The listing builds one solid part. Answer for the finished solid, in the listing's coordinates (mm). A direction names the side the tool comes from. Round coordinates to 2 decimals unless told otherwise and drop trailing zeros. Loops run counter-clockwise (first coordinate to the right, second up) from the corner with the lowest first, then second, coordinate; pieces in that order, holes last. Notation, with made-up numbers: (-31, 29) - (-3, 29) arc R11 ccw to (-3, 40) - close; hole circle Ø10 at (-16.75, -6). An arc over 180 degrees is marked (long way). Write item = value, one per line. Start each with the question number.
1) For a pull along X with two mould halves and no side action, classify faces 4 (the cylindrical face through (24.4, 2.97, 28.21)), 5 (the cylindrical face through (-271.8, 4.9, 56.4)), 6 (the flat face through (-358, 5, 41)), 7 (the flat face through (32, 5, 41)) as released by +X, released by -X, zero draft, split by the parting line, or undercut.
2) Given pin 1 Ø5 at (y, z) = (5, 56) entering from +X, flat-ended and moving along its own axis, determine where the tip first touches the part or whether it passes through.
3) A tool of negligible diameter and unlimited length cuts with its end or side. For faces 1 (the cylindrical face through (24, 5, 59)), 2 (the flat face through (-160, 10, 41)), 3 (the cylindrical face through (-350.4, 4.9, 50.5)), from which of +Z, -Z, +X, -X, +Y, -Y can it reach the whole face along a straight path? Write none if from no direction.
4) Section A-A, the plane x = -200 is taken. Determine the outline of the cut face in (y, z), and give its area (3 significant figures).
5) Section B-B, the plane z = 39 is taken. Determine the outline of the cut face in (x, y).
6) Straight lines are drawn through the part: line 1 along Z through (x, y) = (24.25, 5); line 2 along Z through (x, y) = (-226, 5.25); line 3 along X through (y, z) = (1.5, 24). For each, find the intervals that lie inside material, in ascending order.
Autodesk Inventor part; units mm, degrees
ref_plane "YZ Plane" through (0, 0, 0) normal (1, 0, 0) x (0, 1, 0)
ref_plane "XZ Plane" through (0, 0, 0) normal (0, 1, 0) x (-1, 0, 0)
ref_plane "XY Plane" through (0, 0, 0) normal (0, 0, 1) x (1, 0, 0)
sketch "Boceto1" plane through (0, 0, 0) normal (0, 1, 0) x (-1, 0, 0)
  line L0 (-32, 16) -> (-32, 66)
  line L1 (-32, 66) -> (358, 66)
  line L2 (358, 66) -> (358, 16)
  line L3 (358, 16) -> (-32, 16)
  circle A0 centre (200, 39) radius 7.5
  circle A1 centre (275, 54) radius 4
  circle A2 centre (125, 54) radius 4
  line L4 (179, 60) -> (179, 18)
  line L5 (179, 18) -> (221, 18)
  line L6 (221, 18) -> (221, 60)
  line L7 (221, 60) -> (179, 60)
  circle A3 centre (184.5, 54.5) radius 2
  circle A4 centre (215.5, 54.5) radius 2
  circle A5 centre (215.5, 23.5) radius 2
  circle A6 centre (184.5, 23.5) radius 2
  circle A7 centre (174, 55) radius 2
  line L8 (169, 60) -> (179, 60)
  line L9 (200, 39) -> (195, 39)
  line L10 (195, 39) -> (200, 39)
  line L11 (200, 60) -> (200, 61)
  circle A8 centre (226, 55) radius 2
  line L12 (231, 60) -> (221, 60)
  circle A9 centre (174, 23) radius 2
  line L13 (169, 18) -> (179, 18)
  circle A10 centre (226, 23) radius 2
  line L14 (231, 18) -> (221, 18)
  circle A11 centre (330, 60.5) radius 2
  circle A12 centre (-4, 60.5) radius 2
  point P0 (0, 0)
  dimension "d0" = 50
  dimension "d1" = 390
  dimension "d2" = 15
  dimension "d4" = 8
  dimension "d5" = 8
  dimension "d6" = 15
  dimension "d7" = 75
  dimension "d8" = 75
  dimension "d91" = 4
  dimension "d92" = 4
  dimension "d93" = 4
  dimension "d94" = 4
  dimension "d95" = 31
  dimension "d96" = 31
  dimension "d97" = 31
  dimension "d98" = 31
  dimension "d99" = 5.5
  dimension "d100" = 5.5
  dimension "d101" = 5.5
  dimension "d102" = 5.5
  dimension "d103" = 5.5
  dimension "d104" = 5.5
  dimension "d106" = 4
  dimension "d112" = 5
  dimension "d113" = 5
  dimension "d115" = 42
  dimension "d116" = 12
  dimension "d117" = 12
  dimension "d142" = 4
  dimension "d143" = 4
  dimension "d144" = 5.5
  dimension "d145" = 157
  dimension "d146" = 28
  dimension "d147" = 5.5
  dimension "d148" = 28
extrude "Extrusión1" add sketch "Boceto1" along normal blind 10 contours L0 L1 L2 L3 | L7 L6 L5 L4 | A3 | A4 | A5 | A6
sketch "Boceto6" plane through (32, 0, 66) normal (1, 0, 0) x (0, 0, -1)
  line L0 (0, 0) -> (0, 10)
  line L1 (0, 5) -> (50, 5)
  line L2 (50, 0) -> (50, 10)
  line L3 (50, 5) -> (40, 5)
  line L4 (0, 5) -> (10, 5)
  circle A0 centre (10, 5) radius 3
  circle A1 centre (40, 5) radius 3
  point P0 (66, 0)
  dimension "d35" = 10
  dimension "d36" = 6
  dimension "d37" = 6
  dimension "d119" = 10
hole "Agujero1" at (32, 5, 56) at (32, 5, 26) direction (-1, 0, 0) diameter 6 depth 15 tip angle 118
sketch "Boceto8" plane through (-358, 0, 16) normal (-1, 0, 0) x (0, 0, 1)
  line L0 (50, 0) -> (50, 10)
  line L1 (50, 5) -> (37.5, 5)
  line L2 (37.5, 5) -> (12.5, 5)
  circle A0 centre (40, 5) radius 3
  circle A1 centre (40, 5) radius 3
  circle A2 centre (12.5, 5) radius 3
  point P0 (-16, 0)
  dimension "d58" = 12.5
  dimension "d59" = 25
  dimension "d60" = 6
  dimension "d61" = 6
hole "Agujero3" at (-358, 5, 53.5) at (-358, 5, 28.5) direction (1, 0, 0) diameter 6 depth 15 tip angle 118
thread "Rosca1"
thread "Rosca2"
thread "Rosca3"
thread "Rosca4"
thread "Rosca5"
thread "Rosca6"
thread "Rosca7"
thread "Rosca8"
thread "Rosca9"
thread "Rosca10"
equation "\"d35\" = d119"
properties part number "Culata" material "Aluminio 6061"
Geometry check:
q1.face_4 = zero draft
q1.face_5 = undercut
q1.face_6 = released by -X
q1.face_7 = released by +X
q2.pin_1 = 16.7
q3.face_1 = +X
q3.face_2 = +Z, -Z, +X, -X, +Y
q3.face_3 = -X
q4.outline = (0, 16) - (10, 16) - (10, 31.5) - (0, 31.5) - close; (0, 46.5) - (10, 46.5) - (10, 66) - (0, 66) - close
q4.area = 350 mm2
q5.outline = (-358, 0) - (-207.5, 0) - (-207.5, 10) - (-358, 10) - close; (-192.5, 0) - (32, 0) - (32, 10) - (-192.5, 10) - close
q6.line_1 = 16 to 23, 29 to 53, 59 to 66
q6.line_2 = 16 to 21, 25 to 53, 57 to 66
q6.line_3 = -358 to -227.73, -224.27 to -175.73, -172.27 to 32
